Could you check a few things on this model? Use its own coordinates, in mm. A direction names the side the tool comes from. Give positions to 0.01 mm unless a question says otherwise; leave off trailing zeros. Loops run counter-clockwise (first coordinate to the right, second up) from the corner with the lowest first, then second, coordinate; pieces in that order, holes last. Notation, with made-up numbers: (-11, 24) - (8, 24) arc R24 cw to (8, 37) - close; hole circle Ø8 at (-10, 43). An arc over 180 degrees is marked (long way). Write each question's results on one line, items separated by ' | '. Start each with the question number.
(1) For pin 1 (4 mm diameter, centred on x = -41.42, z = 107.72, fed in from +Y) (3 decimals); pin 2 (1.5 mm diameter, centred on y = 2, z = 7.5, fed in from -X); pin 3 (1.6 mm diameter, centred on y = 1.5, z = 86.5, fed in from -X), each with a flat end and sliding along its axis, tell me the tip position at first contact or that it passes through.
(2) Suppose I cut it at B-B (y = 2.15). Count the separate pieces of the cut face and the enclosed holes in it, and give its area (3 significant figures).
(3) Suppose I cut it at C-C (z = 140). Please give me the cut outline in (x, y) (3 decimals), and give its area (3 significant figures).
(4) Suppose I cut it at D-D (z = 183.5). Please give me the cut outline in (x, y) (3 decimals), and give its area (3 significant figures).
(5) I need wall thicknesses on line 1 (X direction, y = 2, z = 127.5); line 2 (X direction, y = 1.3, z = 196); line 3 (X direction, y = 1.4, z = 7.5). Which ranges of each line are inside material? Lowest first, please.
(6) If we mould it in two halves opening along X, with no side actions, what happens to faces 1 (the face through (-79, 2, -13)), 2 (the face through (-14, 3.175, 74)), 3 (the face through (-57.516, 1.61, 17.041))? For each: released by +X, released by -X, zero draft, split by the parting line, or undercut.
(7) On a 3-axis mill with a long thin cutter (end or side, diameter ignored), from which of +Z, -Z, +X, -X, +Y, -Y can I reach the whole of each face in a straight line? I mean faces 4 (the face through (-24.207, 1.61, 124.636)), 5 (the face through (-50.833, 1.565, 102.084)). Say none if no direction works.
(8) Suppose I cut it at A-A (z = 73). Please give me the cut outline in (x, y) (3 decimals).
from build123d import *

# Parameters (mm, degrees)
SKETCH1_R           = 1.5
SKETCH1_R_2         = 1.65
BOSS_EXTRUDE1_DEPTH = 3.175
SKETCH2_W           = 80
SKETCH2_H           = 15
SKETCH2_R           = 1.5
BOSS_EXTRUDE2_DEPTH = 3.175
FILLET1_R           = 5


with BuildPart() as part:
    # Sketch1 → Boss-Extrude1 (new body)
    with BuildSketch(Plane(origin=(0, 0, 0), x_dir=(1, 0, 0), z_dir=(0, 1, 0))):
        Polygon((-20, -210), (0, -210), (0, 0), (-80, 0), align=None)
        with Locations(Location((-41.422797756, -107.71979577, 0), (0, 0, 270))):
            Circle(SKETCH1_R, mode=Mode.SUBTRACT)
        with Locations(Location((-24.939530082, -165.411232629, 0), (0, 0, 270))):
            Circle(SKETCH1_R, mode=Mode.SUBTRACT)
        with Locations(Location((-10, -195, 0), (0, 0, 270))):
            Circle(SKETCH1_R_2, mode=Mode.SUBTRACT)
        with BuildLine():
            ThreePointArc((-10, -159.75), (-8.5, -161.25), (-10, -162.75))
            ThreePointArc((-10, -162.75), (-11.5, -161.25), (-10, -159.75))
        make_face(mode=Mode.SUBTRACT)
        with BuildLine():
            ThreePointArc((-10, -126), (-8.5, -127.5), (-10, -129))
            ThreePointArc((-10, -129), (-11.5, -127.5), (-10, -126))
        make_face(mode=Mode.SUBTRACT)
        Polygon((-20, -15), (-20, -155.39917583), (-60.114050237, -15), align=None, mode=Mode.SUBTRACT)
        with Locations(Location((-57.90606543, -50.028358912, 0), (0, 0, 270))):
            Circle(SKETCH1_R, mode=Mode.SUBTRACT)
        with Locations(Location((-70.057025119, -7.5, 0), (0, 0, 270))):
            Circle(SKETCH1_R, mode=Mode.SUBTRACT)
        with Locations(Location((-45.028512559, -7.5, 0), (0, 0, 270))):
            Circle(SKETCH1_R, mode=Mode.SUBTRACT)
        with BuildLine():
            ThreePointArc((-10, -92.25), (-8.5, -93.75), (-10, -95.25))
            ThreePointArc((-10, -95.25), (-11.5, -93.75), (-10, -92.25))
        make_face(mode=Mode.SUBTRACT)
        with Locations(Location((-10, -60, 0), (0, 0, 270))):
            Circle(SKETCH1_R_2, mode=Mode.SUBTRACT)
        with Locations(Location((-30, -7.5, 0), (0, 0, 270))):
            Circle(SKETCH1_R, mode=Mode.SUBTRACT)
        with Locations(Location((-10, -7.5, 0), (0, 0, 270))):
            Circle(SKETCH1_R, mode=Mode.SUBTRACT)
    extrude(amount=BOSS_EXTRUDE1_DEPTH)

    # Sketch2 → Boss-Extrude2 (add)
    with BuildSketch(Plane.XZ):
        with Locations((-40, -7.5)):
            Rectangle(SKETCH2_W, SKETCH2_H)
        with Locations(Location((-70.057025119, -7.5, 0), (0, 0, 270))):
            Circle(SKETCH2_R, mode=Mode.SUBTRACT)
        with Locations(Location((-45.028512559, -7.5, 0), (0, 0, 270))):
            Circle(SKETCH2_R, mode=Mode.SUBTRACT)
        with Locations(Location((-10, -7.5, 0), (0, 0, 270))):
            Circle(SKETCH2_R, mode=Mode.SUBTRACT)
    extrude(amount=-BOSS_EXTRUDE2_DEPTH)

    # Fillet1
    fillet1_edges = [part.edges().sort_by_distance(p)[0] for p in [
        (-80, 1.5875, 0),
        (0, 1.5875, 210),
        (-20, 1.5875, 210),
        (-20, 1.5875, 15),
        (-60.114050237, 1.5875, 15),
        (-20, 1.5875, 155.39917583),
        (0, 1.5875, -15),
        (-80, 1.5875, -15),
    ]]
    fillet(fillet1_edges, radius=FILLET1_R)


solid = part.part
Output values:
1) pin 1: y = 3.175 | pin 2: x = -78.07 | pin 3: x = -55.51
2) separate pieces: 1 | enclosed holes: 16 | area: 8,910 mm2
3) outline: (-40, 0) - (0, 0) - (0, 3.175) - (-40, 3.175) - close | area: 127 mm2
4) outline: (-27.571, 0) - (0, 0) - (0, 3.175) - (-27.571, 3.175) - close | area: 87.5 mm2
5) line 1: -43.57 to -11.5, -8.5 to 0 | line 2: -24 to -11.31, -8.69 to 0 | line 3: -77.86 to -71.56, -68.56 to -46.53, -43.53 to -31.5, -28.5 to -11.5, -8.5 to 0
6) face 1: released by -X | face 2: zero draft | face 3: undercut
7) face 4: +Y, -Y | face 5: +Z, -X, +Y, -Y
8) outline: (-59.143, 0) - (-43.543, 0) - (-43.543, 3.175) - (-59.143, 3.175) - close; (-20, 0) - (0, 0) - (0, 3.175) - (-20, 3.175) - close
